Check sheet for the modelled part. Datum: model origin and axes. Units: mm. A direction names the side the tool comes from. Coordinates: 2 decimals unless noted, no trailing zeros. Loops run counter-clockwise (first coordinate to the right, second up) from the corner with the lowest first, then second, coordinate; pieces in that order, holes last. Notation, with made-up numbers: M 37,35.5 L 75,35.5 A8 ccw 75,47.5 Z; hole C 26.25,-5 d7. An arc over 180 degrees is marked long. Answer as CSV lines item,"result". Start each with the question number.
from build123d import *

# Parameters (mm, degrees)
F2_R     = 0.508
F4_W     = 8.763
F4_H     = 1.524
F5_DEPTH = 2.032
F6_W     = 1.016
F6_H     = 5.08
F7_DEPTH = 2.032
F8_R     = 2.3495
F9_DEPTH = 61.722
F10_SIZE = 0.508


with BuildPart() as f1:
    # F0 (on Front) → F1 (revolve)
    with BuildSketch(Plane.XZ):
        with BuildLine():
            ThreePointArc((4.3815, 0), (2.705465, 2.297807), (0, 3.175))
            Line((0, 3.175), (0, 0))
            Line((0, 0), (4.3815, 0))
        make_face()
    revolve(axis=Axis((0, 0, 1.5875), (0, 0, -1)))

    # F2
    f2_edges = [f1.edges().sort_by_distance(p)[0] for p in [
        (-4.3815, 0, 0),
    ]]
    fillet(f2_edges, radius=F2_R)

    # F4 (on plane+point) → F5 (cut)
    with BuildSketch(Plane.XY.offset(3.175)):
        Rectangle(F4_W, F4_H)
    extrude(amount=-F5_DEPTH, mode=Mode.SUBTRACT)

    # F6 (on plane+point) → F7 (cut, through all)
    with BuildSketch(Plane.XY.offset(3.175)):
        Rectangle(F6_W, F6_H)
    extrude(amount=-F7_DEPTH, mode=Mode.SUBTRACT)

    # F8 (on face) → F9 (join)
    with BuildSketch(Plane(origin=(0, 0, 0), x_dir=(1, 0, 0), z_dir=(0, 0, -1))):
        Circle(F8_R)
    extrude(amount=F9_DEPTH)

    # F10
    f10_edges = [f1.edges().sort_by_distance(p)[0] for p in [
        (-2.3495, 0, -61.722),
    ]]
    chamfer(f10_edges, length=F10_SIZE)


solid = f1.part
Item 1: Sectioned sample at A-A, the plane z = -48.5. Record the boundary of the cut face in (x, y).
Item 2: Set-up check for faces 1 (the face through (0.508, -2, 2)), 2 (the face through (-2, -0.762, 2)), 3 (the face through (2, -2, 0)): record each of +Z, -Z, +X, -X, +Y, -Y from which the full face is reachable in a straight line by a thin tool's end or side.
Item 3: Material ranges on line 1 (Y direction, x = 0, z = -10.5); line 2 (Z direction, x = -0.25, y = 0); line 3 (X direction, y = 1, z = -27), recorded low to high. Write a range as from..to.
Item 4: Release check for a two-part mould opening along X. For faces 4 (the face through (2, -0.762, 2)), 5 (the face through (-0.31, -2.33, -30.18)), 6 (the face through (0, 0, 1.143)) record: released by +X, released by -X, zero draft, split by the parting line, or undercut.
Item 5: Go/stop test with flat-tipped pins: pin 1 (1.6 mm diameter, centred on x = -2.5, z = 2.5, fed in from -Y); pin 2 (0.5 mm diameter, centred on y = 2, z = 2, fed in from -X); pin 3 (0.5 mm diameter, centred on y = 2, z = 2.5, fed in from +X). Record where each tip stops, or that it passes through.
Reply:
1,outline,"C 0,0 d4.7"
2,face 1,"+Z"
2,face 2,"+Z, +X, -X"
2,face 3,"-Z"
3,line 1,"-2.35..2.35"
3,line 2,"-61.72..1.14"
3,line 3,"-2.13..2.13"
4,face 4,"zero draft"
4,face 5,"split by the parting line"
4,face 6,"undercut"
5,pin 1,"y = -2.52"
5,pin 2,"x = -2.72"
5,pin 3,"x = 1.98"
